Autodesk Inventor part; units mm, degrees
ref_plane "Plano de trabajo1" through (192.5, 0, 0) normal (1, 0, 0) x (0, 0, -1)
ref_plane "YZ Plane" through (0, 0, 0) normal (1, 0, 0) x (0, 1, 0)
ref_plane "XZ Plane" through (0, 0, 0) normal (0, 1, 0) x (-1, 0, 0)
sketch "Boceto1" plane through (0, 0, 0) normal (1, 0, 0) x (0, 1, 0)
  line L0 (0, 0) -> (0, -220.3761) construction
  arc A0 (0, -155) -> (0, 155) centre (0, 0) ccw
  arc A1 (0, -160) -> (0, 160) centre (0, 0) ccw
  line L1 (0, 155) -> (0, 160) construction
  line L2 (0, -155) -> (0, -160) construction
  line L3 (0, -160) -> (-100, -160)
  line L4 (-100, -160) -> (-100, -155)
  line L5 (-100, -155) -> (0, -155)
  line L6 (0, 155) -> (-100, 155)
  line L7 (-100, 155) -> (-100, 160)
  line L8 (0, 160) -> (-100, 160)
  dimension "d1" = 155
  dimension "d4" = 160
  dimension "d7" = 100
  dimension "d8" = 5
extrude "Extrusión1" add sketch "Boceto1" along normal blind 385
sketch "Boceto2" plane through (0, -100, -160) normal (0, 0, -1) x (-1, 0, 0)
  line L0 (-385, 0) -> (-385, 100) construction
  line L1 (-385, 20) -> (0, 20) construction
  line L2 (0, 0) -> (0, 100) construction
  circle A0 centre (-350, 20) radius 5
  circle A1 centre (-192.5, 20) radius 5
  circle A2 centre (-35, 20) radius 5
  dimension "d9" = 10
  dimension "d10" = 35
  dimension "d11" = 35
  dimension "d14" = 20
extrude "Extrusión2" cut sketch "Boceto2" against normal through all
ref_plane "Plano de trabajo1" through (192.5, 0, 0) normal (1, 0, 0) x (0, 0, -1)
equation "\"Radio_pliegue\" = Grosor"
equation "\"Anchura_desahogo_plegado\" = Grosor"
equation "\"Profundidad_desahogo_plegado\" = 0.5 * Grosor"
equation "\"Radiodetransición\" = Radio_pliegue"
equation "\"Tamaño_de_radio_de_Jacobi\" = Radio_pliegue"
equation "\"TamañoSeparación\" = Grosor"
properties part number "Acrilico" material "Plástico PMMA"
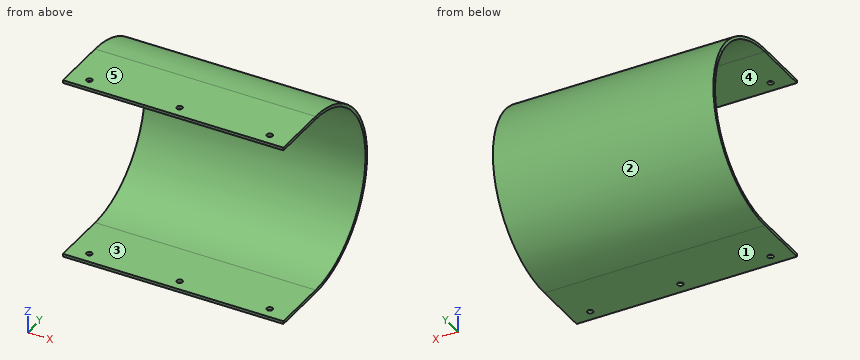
The model under review builds one solid part; all positions refer to its coordinate system, in mm. Face numbers are marked on the shaded views. A direction names the side the tool comes from. Round coordinates to 2 decimals unless told otherwise and drop trailing zeros. Write each loop counter-clockwise with the first axis right and the second up, starting at its lowest first coordinate (ties: lowest second). Pieces come first, ordered by that corner, then holes. Notation, with made-up numbers: (-14, 47) -> (39, 47) arc R11 cw to (39, 53) -> close; hole circle Ø3 at (-39, 67.25). An arc over 180 degrees is marked (long way). Answer as a JSON object with one key per item and string values.
1. Clearance check with flat-ended pins moving along their axes: pin 1 (8 mm diameter, centred on x = 336, z = 52.5, fed in from -Y); pin 2 (12 mm diameter, centred on x = 244, z = -15.5, fed in from -Y); pin 3 (5 mm diameter, centred on x = 205.5, z = -61.5, fed in from +Y). State where each tip first meets the part, or that it passes through.
Results found:
{"pin 1": "stops at y = 144.34", "pin 2": "stops at y = 153.5", "pin 3": "stops at y = 148.72"}
2. To check wall thickness, follow line 1 along Z through (x, y) = (263, -59.5); line 2 along Z through (x, y) = (256.5, 70); line 3 along Y through (x, z) = (320.5, 2). State the ranges of each line that lie inside material, in increasing order.
Results found:
{"line 1": "z = -160 to -155, 155 to 160", "line 2": "z = -143.87 to -138.29, 138.29 to 143.87", "line 3": "y = 154.99 to 159.99"}
3. Machinability: for the marked faces 4 and 5, which of the approach directions +Z, -Z, +X, -X, +Y, -Y give a long, thin tool a straight path to every point of the face, cutting with its end or side? Answer none if there is none.
Results found:
{"face 4": "+X, -X, -Y", "face 5": "+Z, +X, -X, +Y, -Y"}
4. The part is to be moulded in two halves that separate along Z. For the marked faces 1, 2 and 3, say which applies: pulls with the +Z half, pulls with the -Z half, needs draft (parallel to the pull), parting line crosses it, or undercut.
Results found:
{"face 1": "pulls with the -Z half", "face 2": "parting line crosses it", "face 3": "undercut"}
5. We need section C-C on y = -47. State the section outline as (x, z) points, and give its area (3 significant figures).
Results found:
{"outline": "(0, -160) -> (385, -160) -> (385, -155) -> (0, -155) -> close; (0, 155) -> (385, 155) -> (385, 160) -> (0, 160) -> close", "area": "3,850 mm^2"}
6. We need section B-B on x = 35. State the section outline as (y, z) points.
Results found:
{"outline": "(-100, -160) -> (-85, -160) -> (-85, -155) -> (-100, -155) -> close; (-100, 155) -> (-85, 155) -> (-85, 160) -> (-100, 160) -> close; (-75, -160) -> (0, -160) arc R160 ccw to (0, 160) -> (-75, 160) -> (-75, 155) -> (0, 155) arc R155 cw to (0, -155) -> (-75, -155) -> close"}
7. We need section A-A on y = -80. State how many separate pieces and enclosed holes the cut face has, and give its area (3 significant figures).
Results found:
{"separate pieces": "8", "enclosed holes": "0", "area": "3,550 mm^2"}
8. We need section D-D on y = 135. State the section outline as (x, z) points.
Results found:
{"outline": "(0, -85.88) -> (385, -85.88) -> (385, -76.16) -> (0, -76.16) -> close; (0, 76.16) -> (385, 76.16) -> (385, 85.88) -> (0, 85.88) -> close"}
